Here's the drawing with two shaded views (mm, measured from the low corner). I have some questions. A direction names the side the tool comes from. Coordinates: 2 decimals unless noted, no trailing zeros. Write each loop counter-clockwise with the first axis right and the second up, starting at its lowest first coordinate (ties: lowest second). Pieces come first, ordered by that corner, then holes.
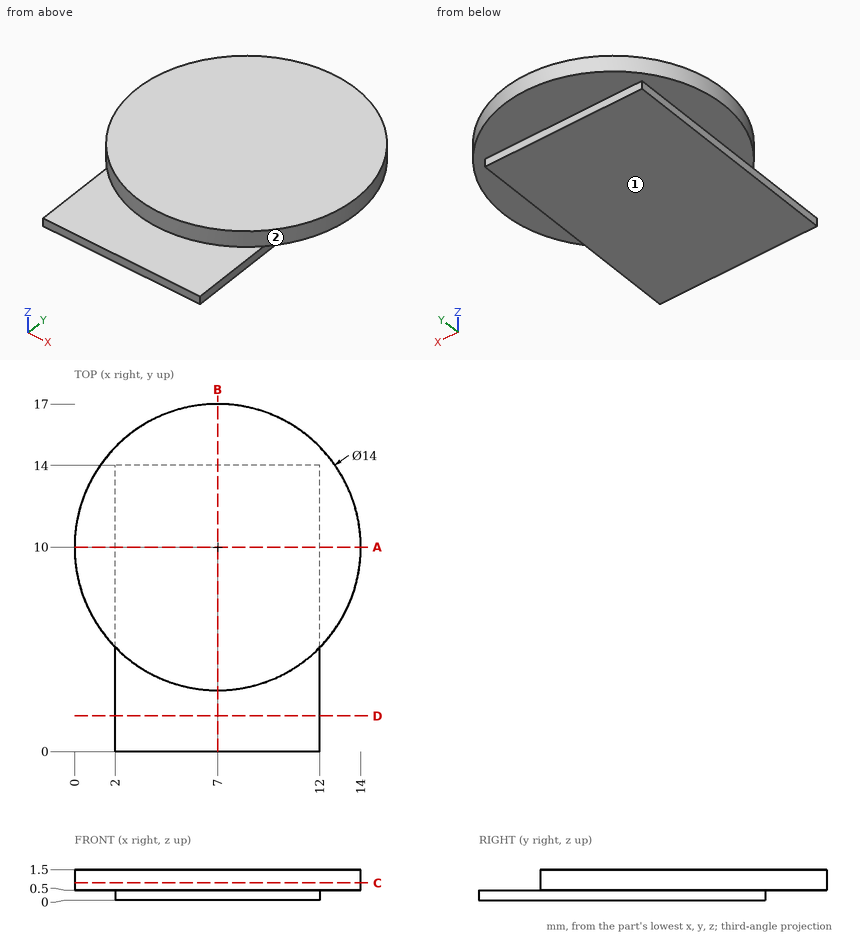
1. I want a section at D-D on y = 1.75. Please give me the cut outline in (x, z).
Verdict:
outline: (2, 0) - (12, 0) - (12, 0.5) - (2, 0.5) - close
2. Please list where these lines run through material, in increasing order: line 1 along Z through (x, y) = (4, 1.25); line 2 along Z through (x, y) = (1, 12.25); line 3 along X through (y, z) = (4.5, 0.25).
Verdict:
line 1: z = 0 to 0.5
line 2: z = 0.5 to 1.5
line 3: x = 2 to 12
3. I want a section at A-A on y = 10. Please give me the cut outline in (x, z), plus the area to 3 significant figures.
Verdict:
outline: (0, 0.5) - (2, 0.5) - (2, 0) - (12, 0) - (12, 0.5) - (14, 0.5) - (14, 1.5) - (0, 1.5) - close
area: 19.0 mm2
4. I want a section at C-C on z = 0.85. Please give me the cut outline in (x, y).
Verdict:
outline: circle Ø14 at (7, 10)
5. On a 3-axis mill with a long thin cutter (end or side, diameter ignored), from which of +Z, -Z, +X, -X, +Y, -Y can I reach the whole of each face in a straight line? I mean the marked faces 1 and 2. Say none if no direction works.
Verdict:
face 1: -Z, +X, -X, +Y, -Y
face 2: +Z
6. I want a section at B-B on x = 7. Please give me the cut outline in (y, z), plus the area to 3 significant figures.
Verdict:
outline: (0, 0) - (14, 0) - (14, 0.5) - (17, 0.5) - (17, 1.5) - (3, 1.5) - (3, 0.5) - (0, 0.5) - close
area: 21.0 mm2
7. For pin 1 (1.5 mm diameter, centred on x = 7, y = 1.5, fed in from +Z); pin 2 (0.6 mm diameter, centred on y = 10.5, z = 0, fed in from +X), each with a flat end and sliding along its axis, tell me the tip position at first contact or that it passes through.
Verdict:
pin 1: stops at z = 0.5
pin 2: stops at x = 12
